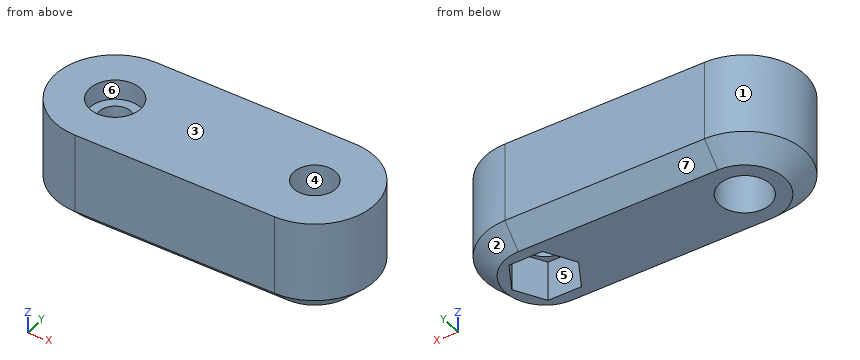
from build123d import *

# Parameters (mm, degrees)
EXTRUDE_1_DEPTH     = 10
CHAMFER_1_SIZE      = 2
CUT_EXTRUDE_1_DEPTH = 4


with BuildPart() as part:
    # 草图1 → 凸台-拉伸1 (new body)
    with BuildSketch(Plane.XY):
        with BuildLine():
            Line((0, 6), (20, 6))
            ThreePointArc((20, 6), (26, 0), (20, -6))
            Line((20, -6), (0, -6))
            ThreePointArc((0, -6), (-6, 0), (0, 6))
        make_face()
    extrude(amount=EXTRUDE_1_DEPTH)

    # 草图2 → 切除-旋转1 (revolve, cut)
    with BuildSketch(Plane(origin=(0, 0, 0), x_dir=(1, 0, 0), z_dir=(0, 1, 0))):
        Polygon((0, 0), (-2.55, 0), (-2.55, -5), (-1.6, -5), (-1.6, -8), (-2.55, -8), (-2.55, -10), (0, -10), align=None)
    revolve(axis=Axis((0, 0, 10), (0, 0, -1)), mode=Mode.SUBTRACT)

    # 草图3 → 切除-旋转2 (revolve, cut)
    with BuildSketch(Plane(origin=(0, 0, 0), x_dir=(1, 0, 0), z_dir=(0, 1, 0))):
        Polygon((20, 0), (17.42, 0), (17.42, -5), (17.9, -5), (17.9, -10), (20, -10), align=None)
    revolve(axis=Axis((20, 0, 10), (0, 0, -1)), mode=Mode.SUBTRACT)

    # 倒角1
    chamfer_1_edges = [part.edges().sort_by_distance(p)[0] for p in [
        (10, 6, 0),
        (26, 0, 0),
        (10, -6, 0),
        (-6, 0, 0),
    ]]
    chamfer(chamfer_1_edges, length=CHAMFER_1_SIZE)

    # 草图4 → 切除-拉伸1 (cut)
    with BuildSketch(Plane(origin=(0, 0, 0), x_dir=(-1, 0, 0), z_dir=(0, 0, -1))):
        Polygon((-23.348631561, 0), (-21.674315781, -2.9), (-18.325684219, -2.9), (-16.651368439, 0), (-18.325684219, 2.9), (-21.674315781, 2.9), align=None)
    extrude(amount=-CUT_EXTRUDE_1_DEPTH, mode=Mode.SUBTRACT)


solid = part.part
Verification items for the finished model (mm, model axes). Face numbers are marked on the shaded views. A direction names the side the tool comes from. Coordinates: 2 decimals unless noted, no trailing zeros. Order: outer loops, then holes, each group sorted by start corner. A loop starts at its lowest first (then second) coordinate and runs counter-clockwise, first axis right, second up. Notation, with made-up numbers: M 84.5,55.5 L 139.5,55.5 A18 cw 139.5,64.5 Z; hole C -30,12.5 d3. An arc over 180 degrees is marked long. Return JSON: item names as keys, results as strings.
1) Gauge pin test, flat ends, axial feed: pin 1 (2 mm diameter, centred on y = -3.5, z = 2, fed in from -X); pin 2 (5.5 mm diameter, centred on x = 20, y = 0, fed in from -Z); pin 3 (4.5 mm diameter, centred on x = 0, y = 0, fed in from +Z). Record the tip position at first contact, or that the pin passes through.
Answer list:
{"pin 1": "x = -5.45", "pin 2": "z = 4", "pin 3": "z = 8"}
2) Cross-section at C-C, the plane z = 7.5. Record the boundary of the cut face in (x, y).
Answer list:
{"outline": "M 0,-6 L 20,-6 A6 ccw 20,6 L 0,6 A6 ccw Z; hole C 0,0 d3.2; hole C 20,0 d4.2"}
3) Release check for a two-part mould opening along X. For the marked faces 1, 2, 3 and 4 record: +X half, -X half, draft (parallel to the pull), parting line (faces both ways), or undercut.
Answer list:
{"face 1": "-X half", "face 2": "+X half", "face 3": "draft", "face 4": "undercut"}
4) Thickness scan on L1, parallel to Y at x = 0, z = 7.3; L2, parallel to Y at x = 20, z = 4.65; L3, parallel to X at y = 2.5, z = 5.5. Record the ranges inside material, lowest first. Write a range as [from, to].
Answer list:
{"L1": "[-6, -1.6], [1.6, 6]", "L2": "[-6, -2.58], [2.58, 6]", "L3": "[-5.45, 25.45]"}
5) Cross-section at B-B, the plane y = -1. Count the separate pieces of the cut face and the enclosed holes in it, and give its area (3 significant figures).
Answer list:
{"separate pieces": "3", "enclosed holes": "0", "area": "229 mm2"}
6) Access from +Z, -Z, +X, -X, +Y, -Y to the whole of each face (thin tool, end or side, straight path). Record for the marked faces 5, 6 and 7.
Answer list:
{"face 5": "-Z", "face 6": "+Z", "face 7": "-Z, +X, -X, +Y"}
7) Cross-section at A-A, the plane z = 8.75. Record the boundary of the cut face in (x, y), and give its area (3 significant figures).
Answer list:
{"outline": "M 0,-6 L 20,-6 A6 ccw 20,6 L 0,6 A6 ccw Z; hole C 0,0 d5.1; hole C 20,0 d4.2", "area": "319 mm2"}
